Geometry check sheet. Reference: the model listing, model coordinates, mm. A direction names the side the tool comes from. Give positions to 0.01 mm unless a question says otherwise; leave off trailing zeros. Order: outer loops, then holes, each group sorted by start corner. A loop starts at its lowest first (then second) coordinate and runs counter-clockwise, first axis right, second up.
from build123d import *

# Parameters (mm, degrees)
EXTRUDE_1_DEPTH          = 2.5
SKETCH_1_4_R             = 3
EXTRUDE_2_DEPTH          = 3
CUT_EXTRUDE_1_DEPTH      = 51.090903435
CUT_EXTRUDE_1_DEPTH_BACK = 51.090903435
SKETCH_1_3_R             = 2
FILLET_1_R               = 3
EXTRUDE_START            = -2.5
SKETCH_2_R               = 2
EXTRUDE_3_DEPTH          = 2.5
SKETCH_2_3_R             = 1.8
EXTRUDE_4_DEPTH          = 1.5
EXTRUDE_6_DEPTH          = 2.5
EXTRUDE_START_2          = -7
EXTRUDE_5_DEPTH          = 7
FILLET_3_R               = 10
SKETCH_5_R               = 0.25
CUT_EXTRUDE_2_DEPTH      = 2


with BuildPart() as part:
    # 草图1 → 凸台-拉伸1 (new body)
    with BuildSketch(Plane(origin=(0, 0, 0), x_dir=(0, 0, -1), z_dir=(1, 0, 0))):
        with BuildLine():
            Line((40.737143614, 0), (0, 0))
            Line((0, 0), (2.48051592, -3.542543867))
            ThreePointArc((2.48051592, -3.542543867), (4.165783411, -4.487079684), (5.367176995, -6))
            Line((5.367176995, -6), (44.201245229, -6))
            ThreePointArc((44.201245229, -6), (40.737143614, -4), (40.737143614, 0))
        make_face()
        with BuildLine():
            Line((2.48051592, -3.542543867), (0, 0))
            Line((0, 0), (-2.681672007, 3.829824531))
            ThreePointArc((-2.681672007, 3.829824531), (-4.811127311, -0.102785303), (-9.234888361, -0.758786959))
            Line((-9.234888361, -0.758786959), (-4.072700434, -8.131155358))
            ThreePointArc((-4.072700434, -8.131155358), (-1.94324513, -4.198545524), (2.48051592, -3.542543867))
        make_face()
        with BuildLine():
            ThreePointArc((48.201245229, -2), (45.23652141, 1.863703305), (40.737143614, 0))
            Line((40.737143614, 0), (44.201245229, 0))
            ThreePointArc((44.201245229, 0), (45.615458792, -0.585786438), (46.201245229, -2))
            ThreePointArc((46.201245229, -2), (45.615458792, -3.414213562), (44.201245229, -4))
            Line((44.201245229, -4), (44.201245229, -6))
            ThreePointArc((44.201245229, -6), (47.029672354, -4.828427125), (48.201245229, -2))
        make_face()
        with BuildLine():
            Line((44.201245229, 0), (40.737143614, 0))
            ThreePointArc((40.737143614, 0), (40.737143614, -4), (44.201245229, -6))
            Line((44.201245229, -6), (44.201245229, -4))
            ThreePointArc((44.201245229, -4), (42.201245229, -2), (44.201245229, 0))
        make_face()
        with BuildLine():
            ThreePointArc((5.367176995, -6), (4.165783411, -4.487079684), (2.48051592, -3.542543867))
            Line((2.48051592, -3.542543867), (4.201245229, -6))
            Line((4.201245229, -6), (5.367176995, -6))
        make_face()
        with BuildLine():
            Line((4.201245229, -6), (2.48051592, -3.542543867))
            ThreePointArc((2.48051592, -3.542543867), (-1.94324513, -4.198545524), (-4.072700434, -8.131155358))
            Line((-4.072700434, -8.131155358), (-2.351971125, -10.588611491))
            Line((-2.351971125, -10.588611491), (-1.532819081, -10.015035054))
            ThreePointArc((-1.532819081, -10.015035054), (-0.796092257, -5.836849613), (3.382093185, -6.573576436))
            Line((3.382093185, -6.573576436), (4.201245229, -6))
        make_face()
        with BuildLine():
            ThreePointArc((-9.234888361, -0.758786959), (-4.811127311, -0.102785303), (-2.681672007, 3.829824531))
            Line((-2.681672007, 3.829824531), (-4.402401316, 6.287280664))
            Line((-4.402401316, 6.287280664), (-6.040705405, 5.140127792))
            ThreePointArc((-6.040705405, 5.140127792), (-5.771575592, 4.594386518), (-5.679009493, 3.992974919))
            ThreePointArc((-5.679009493, 3.992974919), (-7.077597894, 2.085541017), (-9.317313582, 2.845822046))
            Line((-9.317313582, 2.845822046), (-10.95561767, 1.698669174))
            Line((-10.95561767, 1.698669174), (-9.234888361, -0.758786959))
        make_face()
        with BuildLine():
            Line((-4.402401316, 6.287280664), (-2.681672007, 3.829824531))
            ThreePointArc((-2.681672007, 3.829824531), (-2.679675166, 3.911388863), (-2.679009493, 3.992974919))
            ThreePointArc((-2.679009493, 3.992974919), (-10.613341245, 8.041394014), (-9.234888361, -0.758786959))
            Line((-9.234888361, -0.758786959), (-10.95561767, 1.698669174))
            Line((-10.95561767, 1.698669174), (-9.317313582, 2.845822046))
            ThreePointArc((-9.317313582, 2.845822046), (-8.826162366, 5.631279008), (-6.040705405, 5.140127792))
            Line((-6.040705405, 5.140127792), (-4.402401316, 6.287280664))
        make_face()
        with BuildLine():
            ThreePointArc((46.201245229, -2), (45.615458792, -0.585786438), (44.201245229, 0))
            Line((44.201245229, 0), (44.201245229, -4))
            ThreePointArc((44.201245229, -4), (45.615458792, -3.414213562), (46.201245229, -2))
        make_face()
        with BuildLine():
            Line((44.201245229, -4), (44.201245229, 0))
            ThreePointArc((44.201245229, 0), (42.201245229, -2), (44.201245229, -4))
        make_face()
        with BuildLine():
            Line((5.367176995, -6), (4.201245229, -6))
            Line((4.201245229, -6), (3.382093185, -6.573576436))
            ThreePointArc((3.382093185, -6.573576436), (3.785787904, -7.392188347), (3.924637052, -8.294305745))
            ThreePointArc((3.924637052, -8.294305745), (1.826754451, -11.155456598), (-1.532819081, -10.015035054))
            Line((-1.532819081, -10.015035054), (-2.351971125, -10.588611491))
            Line((-2.351971125, -10.588611491), (-4.072700434, -8.131155358))
            ThreePointArc((-4.072700434, -8.131155358), (0.843050996, -13.293640073), (5.924637052, -8.294305745))
            ThreePointArc((5.924637052, -8.294305745), (5.783273678, -7.113776143), (5.367176995, -6))
        make_face()
        with BuildLine():
            ThreePointArc((3.924637052, -8.294305745), (3.785787904, -7.392188347), (3.382093185, -6.573576436))
            Line((3.382093185, -6.573576436), (2.562941141, -7.147152873))
            ThreePointArc((2.562941141, -7.147152873), (2.832070954, -7.692894146), (2.924637052, -8.294305745))
            ThreePointArc((2.924637052, -8.294305745), (1.526048651, -10.201739647), (-0.713667036, -9.441458618))
            Line((-0.713667036, -9.441458618), (-1.532819081, -10.015035054))
            ThreePointArc((-1.532819081, -10.015035054), (1.826754451, -11.155456598), (3.924637052, -8.294305745))
        make_face()
        with BuildLine():
            Line((2.562941141, -7.147152873), (3.382093185, -6.573576436))
            ThreePointArc((3.382093185, -6.573576436), (-0.796092257, -5.836849613), (-1.532819081, -10.015035054))
            Line((-1.532819081, -10.015035054), (-0.713667036, -9.441458618))
            ThreePointArc((-0.713667036, -9.441458618), (-0.222515821, -6.656001657), (2.562941141, -7.147152873))
        make_face()
        with BuildLine():
            ThreePointArc((-5.679009493, 3.992974919), (-5.771575592, 4.594386518), (-6.040705405, 5.140127792))
            Line((-6.040705405, 5.140127792), (-9.317313582, 2.845822046))
            ThreePointArc((-9.317313582, 2.845822046), (-7.077597894, 2.085541017), (-5.679009493, 3.992974919))
        make_face()
        with BuildLine():
            Line((-9.317313582, 2.845822046), (-6.040705405, 5.140127792))
            ThreePointArc((-6.040705405, 5.140127792), (-8.826162366, 5.631279008), (-9.317313582, 2.845822046))
        make_face()
        with BuildLine():
            ThreePointArc((2.924637052, -8.294305745), (2.832070954, -7.692894146), (2.562941141, -7.147152873))
            Line((2.562941141, -7.147152873), (-0.713667036, -9.441458618))
            ThreePointArc((-0.713667036, -9.441458618), (1.526048651, -10.201739647), (2.924637052, -8.294305745))
        make_face()
        with BuildLine():
            Line((-0.713667036, -9.441458618), (2.562941141, -7.147152873))
            ThreePointArc((2.562941141, -7.147152873), (-0.222515821, -6.656001657), (-0.713667036, -9.441458618))
        make_face()
    extrude(amount=EXTRUDE_1_DEPTH)

    # 草图1<4> → 凸台-拉伸2 (add)
    with BuildSketch(Plane(origin=(0, 0, 0), x_dir=(0, 0, -1), z_dir=(1, 0, 0))):
        with Locations((0.924637052, -8.294305745)):
            Circle(SKETCH_1_4_R)
    extrude(amount=-EXTRUDE_2_DEPTH)

    # 草图1<3> → 切除-拉伸1 (cut, two sides: drawn at the far end of the back side and taken through both)
    with BuildSketch(Plane(origin=(0, 0, 0), x_dir=(0, 0, -1), z_dir=(1, 0, 0)).offset(-CUT_EXTRUDE_1_DEPTH_BACK)):
        with Locations((-7.679009493, 3.992974919)):
            Circle(SKETCH_1_3_R)
        with Locations((44.201245229, -2)):
            Circle(SKETCH_1_3_R)
        with Locations((0.924637052, -8.294305745)):
            Circle(SKETCH_1_3_R)
    extrude(amount=CUT_EXTRUDE_1_DEPTH + CUT_EXTRUDE_1_DEPTH_BACK, mode=Mode.SUBTRACT)

    # 圆角1
    fillet_1_edges = [part.edges().sort_by_distance(p)[0] for p in [
        (1.25, -6, -5.367176995),
        (1.25, 0, 0),
        (1.25, 0, -40.737143614),
        (1.25, -0.758786959, 9.234888361),
        (1.25, -8.131155358, 4.072700434),
    ]]
    fillet(fillet_1_edges, radius=FILLET_1_R)

    # 草图2 → 凸台-拉伸3 (add)
    with BuildSketch(Plane(origin=(2.5, 0, 0), x_dir=(0, 0, -1), z_dir=(1, 0, 0)).offset(EXTRUDE_START)):
        with Locations((-7.679009493, 3.992974919)):
            Circle(SKETCH_2_R)
    extrude(amount=EXTRUDE_3_DEPTH)

    # 草图2<3> → 凸台-拉伸4 (add)
    with BuildSketch(Plane(origin=(2.5, 0, 0), x_dir=(0, 0, -1), z_dir=(1, 0, 0))):
        with Locations((-7.679009493, 3.992974919)):
            Circle(SKETCH_2_3_R)
    extrude(amount=EXTRUDE_4_DEPTH)

    # 草图4 → 凸台-拉伸6 (add)
    with BuildSketch(Plane(origin=(2.5, 0, 0), x_dir=(0, 0, -1), z_dir=(1, 0, 0))):
        Polygon((-5.244772745, 8.360410259), (9.755227255, 0), (-5.244772745, 0), align=None)
    extrude(amount=-EXTRUDE_6_DEPTH)

    # 草图3 → 凸台-拉伸5 (add)
    with BuildSketch(Plane(origin=(2.5, 0, 0), x_dir=(0, 0, -1), z_dir=(1, 0, 0)).offset(EXTRUDE_START_2)):
        with BuildLine():
            Line((-12.894335644, 6.959517206), (-12.261585188, 5.992974919))
            ThreePointArc((-12.261585188, 5.992974919), (-10.417622281, 8.176275052), (-7.679009493, 8.992974919))
            Line((-7.679009493, 8.992974919), (-8.311759949, 9.959517206))
            ThreePointArc((-8.311759949, 9.959517206), (-10.965344838, 9.012935078), (-12.894335644, 6.959517206))
        make_face()
    extrude(amount=EXTRUDE_5_DEPTH)

    # 圆角3
    fillet_3_edges = [part.edges().sort_by_distance(p)[0] for p in [
        (1.25, 0, -9.755227255),
    ]]
    fillet(fillet_3_edges, radius=FILLET_3_R)

    # 镜向1: part across plane


with BuildPart() as part_1:
    add(part.part)
    add(part.part.mirror(Plane.ZY.offset(4.5)))

    # 草图5 → 切除-拉伸2 (cut)
    with BuildSketch(Plane(origin=(4, 0, 0), x_dir=(0, 0, -1), z_dir=(1, 0, 0))):
        with Locations((-7.679009493, 3.992974919)):
            Circle(SKETCH_5_R)
    extrude(amount=-CUT_EXTRUDE_2_DEPTH, mode=Mode.SUBTRACT)


solid = part_1.part
Item 1: Gauge pin test, flat ends, axial feed: pin 1 (11 mm diameter, centred on y = 3, z = -5.5, fed in from +X); pin 2 (0.6 mm diameter, centred on y = 4, z = 7.5, fed in from +X); pin 3 (5 mm diameter, centred on x = -7.5, y = 2.5, fed in from -Z); pin 4 (10 mm diameter, centred on y = 2.5, z = -5.5, fed in from -X). Record the tip position at first contact, or that the pin passes through.
Reported:
pin 1: stops at x = 2.5
pin 2: stops at x = 4
pin 3: stops at z = -47.32
pin 4: stops at x = -11.5
Item 2: Sectioned sample at A-A (z = -31.5). Enter the section's corners in (x, y).
Reported:
outline: (-11.5, -6) - (-9, -6) - (-9, 0) - (-11.5, 0) - close; (0, -6) - (2.5, -6) - (2.5, 0) - (0, 0) - close
Item 3: Sectioned sample at C-C (x = -5.25). Enter the section's corners in (y, z), and give its area (3 significant figures).
Reported:
outline: (5.99, 12.26) arc R5 cw to (8.99, 7.68) - (9.96, 8.31) arc R6 ccw to (6.96, 12.89) - close
area: 5.74 mm2
Item 4: Sectioned sample at B-B (x = 1.25). Give the number of separate pieces and of enclosed holes in the cut face, and give its area (3 significant figures).
Reported:
separate pieces: 1
enclosed holes: 2
area: 510 mm2
Item 5: Scan lines: L1, parallel to X at y = 4.5, z = 0; L2, parallel to Y at x = -9.5, z = -23; L3, parallel to Z at x = -10.7, y = -2. Record each from-to range of solid material in increasing order.
Reported:
L1: x = -11.5 to -9, 0 to 2.5
L2: y = -6 to 0
L3: z = -48.2 to -46.2, -42.2 to 8.37
Item 6: Set-up check for faces 5 (the cylindrical face through (-7.52, -5.32, -0.53)), 6 (the cylindrical face through (1.268, 0.216, -40.421)), 7 (the flat face through (-10, -6, -26)): record each of +Z, -Z, +X, -X, +Y, -Y from which the full face is reachable in a straight line by a thin tool's end or side.
Reported:
face 5: none
face 6: +X, -X, +Y
face 7: -Z, +X, -X, -Y
Item 7: Draft check along Z on faces 1 (the cylindrical face through (-10.233, -2.766, -46.049)), 2 (the flat face through (-9, -1, -11)), 3 (the cylindrical face through (-10.268, -8.075, 4.225)), 4 (the cylindrical face through (-10.268, 0.216, -40.421)). Enter one of: released by +Z, released by -Z, zero draft, split by the parting line, or undercut.
Reported:
face 1: undercut
face 2: zero draft
face 3: released by +Z
face 4: undercut
